Source: CAD feature listing. Evaluate the final solid. Frame: model axes, mm. A direction names the side the tool comes from. Coordinates: 2 decimals unless noted, no trailing zeros. Write each loop counter-clockwise with the first axis right and the second up, starting at its lowest first coordinate (ties: lowest second). Pieces come first, ordered by that corner, then holes. Notation, with made-up numbers: M -29,16.5 L 21,16.5 A29 cw 21,51.5 Z; hole C 22.5,4.25 d4. An arc over 180 degrees is marked long. Answer as CSV lines item,"result". Start each with the question number.
1. Reachability of faces 1 (the face through (-12.035, -22.785, -3.199)), 2 (the face through (-2.38, -10.74, -0.05)), 3 (the face through (11.89, -23.03, 0.04)) from +Z, -Z, +X, -X, +Y, -Y: full face, straight path, thin tool, end or side. Return the list, or none.
2. Section A-A on x = 0. Return the cut outline in (y, z).
3. Contact query for flat-ended pins moving along their axis: pin 1 Ø3 at (y, z) = (-10.5, -2.5) entering from -X; pin 2 Ø13 at (x, y) = (-25.98, -15) entering from +Z; pin 3 Ø1.5 at (y, z) = (24, -1) entering from -X; pin 4 Ø1.5 at (y, z) = (11, 2.5) entering from +X. Output: stop coordinate, or through.
4. Line query: probe 1 along Y at (x, z) = (0, 0.2); probe 2 along Y at (x, z) = (4.5, 1.25); probe 3 along Y at (x, z) = (26.5, 0.25). Output: solid intervals per line, ascending. Write a range as [from, to].
5. Mould query, pull axis Y, two halves, no side actions, for faces 4 (the face through (26, 1, 3)), 5 (the face through (12.231, -22.898, 3.199)), 6 (the face through (36.142, -19.213, -0.049)). Classes: pulls with the +Y half, pulls with the -Y half, needs draft (parallel to the pull), parting line crosses it, or undercut.
6. Section B-B on y = -5. Count the separate pieces of the cut face and the enclosed holes in it, plus the area to 3 significant figures.
```python
from build123d import *

# Parameters (mm, degrees)
F0_R     = 11
F1_DEPTH = 3.5
F2_R     = 1
F3_R     = 1


with BuildPart() as f1:
    # F0 (on Top) → F1 (new body, symmetric)
    with BuildSketch(Plane.XY):
        with BuildLine():
            ThreePointArc((-32.980762, -2.875644), (-38.105118, -22), (-18.980762, -27.124356))
            Line((-18.980762, -27.124356), (-5, -19.052559))
            ThreePointArc((-5, -19.052559), (0, -17.712813), (5, -19.052559))
            Line((5, -19.052559), (18.980762, -27.124356))
            ThreePointArc((18.980762, -27.124356), (38.105118, -22), (32.980762, -2.875644))
            Line((32.980762, -2.875644), (19, 5.196152))
            ThreePointArc((19, 5.196152), (15.339746, 8.856406), (14, 13.856406))
            Line((14, 13.856406), (14, 30))
            ThreePointArc((14, 30), (0, 44), (-14, 30))
            Line((-14, 30), (-14, 13.856406))
            ThreePointArc((-14, 13.856406), (-15.339746, 8.856406), (-19, 5.196152))
            Line((-19, 5.196152), (-32.980762, -2.875644))
        make_face()
        with Locations((-25.980762, -15)):
            Circle(F0_R, mode=Mode.SUBTRACT)
        Circle(F0_R, mode=Mode.SUBTRACT)
        with Locations((25.980762, -15)):
            Circle(F0_R, mode=Mode.SUBTRACT)
        with Locations((0, 30)):
            Circle(F0_R, mode=Mode.SUBTRACT)
    extrude(amount=F1_DEPTH, both=True)

    # F2
    f2_edges = [f1.edges().sort_by_distance(p)[0] for p in [
        (0, 44, 3.5),
        (14, 21.928203, 3.5),
        (15.339746, 8.856406, 3.5),
        (25.990381, 1.160254, 3.5),
        (38.105118, -22, 3.5),
        (11.990381, -23.088457, 3.5),
        (0, -17.712813, 3.5),
        (-11.990381, -23.088457, 3.5),
        (-38.105118, -22, 3.5),
        (-25.990381, 1.160254, 3.5),
        (-15.339746, 8.856406, 3.5),
        (-14, 21.928203, 3.5),
    ]]
    fillet(f2_edges, radius=F2_R)

    # F3
    f3_edges = [f1.edges().sort_by_distance(p)[0] for p in [
        (-11.990381, -23.088457, -3.5),
        (-38.105118, -22, -3.5),
        (-25.990381, 1.160254, -3.5),
        (-15.339746, 8.856406, -3.5),
        (-14, 21.928203, -3.5),
        (-11, 30, -3.5),
        (14, 21.928203, -3.5),
        (15.339746, 8.856406, -3.5),
        (25.990381, 1.160254, -3.5),
        (38.105118, -22, -3.5),
        (11.990381, -23.088457, -3.5),
        (0, -17.712813, -3.5),
    ]]
    fillet(f3_edges, radius=F3_R)


solid = f1.part
```
Values:
1,face 1,"-Z, -Y"
1,face 2,"+Z, -Z"
1,face 3,"+Z, -Z, -Y"
2,outline,"M -17.71,-2.5 A1 ccw -16.71,-3.5 L -11,-3.5 L -11,3.5 L -16.71,3.5 A1 ccw -17.71,2.5 Z; M 11,-3.5 L 18,-3.5 A1 ccw 19,-2.5 L 19,3.5 L 11,3.5 Z; M 41,-2.5 A1 ccw 42,-3.5 L 43,-3.5 A1 ccw 44,-2.5 L 44,2.5 A1 ccw 43,3.5 L 41,3.5 Z"
3,pin 1,"x = -39.66"
3,pin 2,"through"
3,pin 3,"x = -14"
3,pin 4,"x = 14.67"
4,probe 1,"[-17.71, -11], [11, 19], [41, 44]"
4,probe 2,"[-18.78, -10.04], [10.04, 19.96], [40.04, 43.26]"
4,probe 3,"[-28.99, -25.99], [-4.01, 0.87]"
5,face 4,"pulls with the +Y half"
5,face 5,"pulls with the -Y half"
5,face 6,"undercut"
6,separate pieces,"4"
6,enclosed holes,"0"
6,area,"234 mm²"
